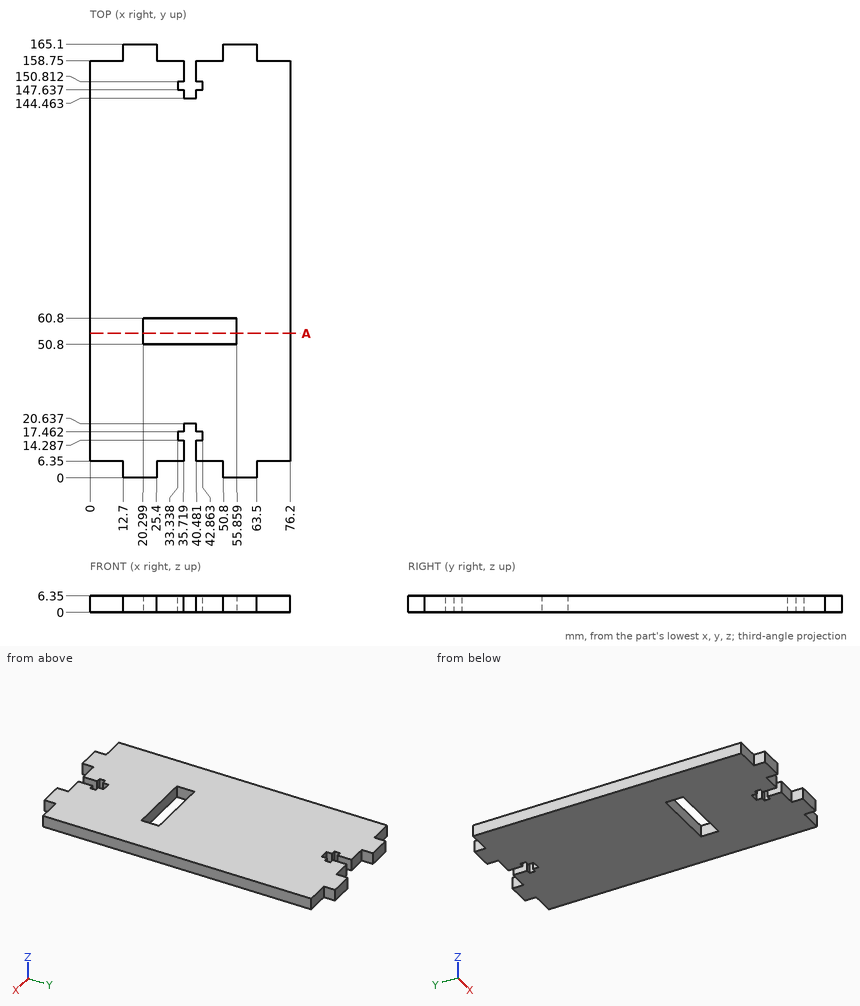
Here's the drawing with two shaded views (mm, measured from the low corner). I have some questions. Coordinates: 2 decimals unless noted, no trailing zeros. Order: outer loops, then holes, each group sorted by start corner. A loop starts at its lowest first (then second) coordinate and runs counter-clockwise, first axis right, second up.
Item 1: If we section it at A-A, the plane y = 55: List the corners of the cut face in (x, z) for me.
Response values:
outline: (0, 0) - (20.3, 0) - (20.3, 6.35) - (0, 6.35) - close; (55.86, 0) - (76.2, 0) - (76.2, 6.35) - (55.86, 6.35) - close
Item 2: I need wall thicknesses on probe 1 along Y at (x, z) = (41, 5.5); probe 2 along X at (y, z) = (56, 0.75); probe 3 along Y at (x, z) = (38, 5.5). Which ranges of each line are inside material? Lowest first, please.
Response values:
probe 1: y = 6.35 to 14.29, 17.46 to 50.8, 60.8 to 147.64, 150.81 to 158.75
probe 2: x = 0 to 20.3, 55.86 to 76.2
probe 3: y = 20.64 to 50.8, 60.8 to 144.46
Item 3: I'm going to push flat-ended pins straight in: pin 1 Ø3 at (x, z) = (72, 3) entering from +Y; pin 2 Ø1.9 at (y, z) = (3.5, 2.5) entering from -X; pin 3 Ø1.9 at (y, z) = (4.5, 4.5) entering from +X. Where does each tip first touch, or does it pass through?
Response values:
pin 1: stops at y = 158.75
pin 2: stops at x = 12.7
pin 3: stops at x = 63.5
